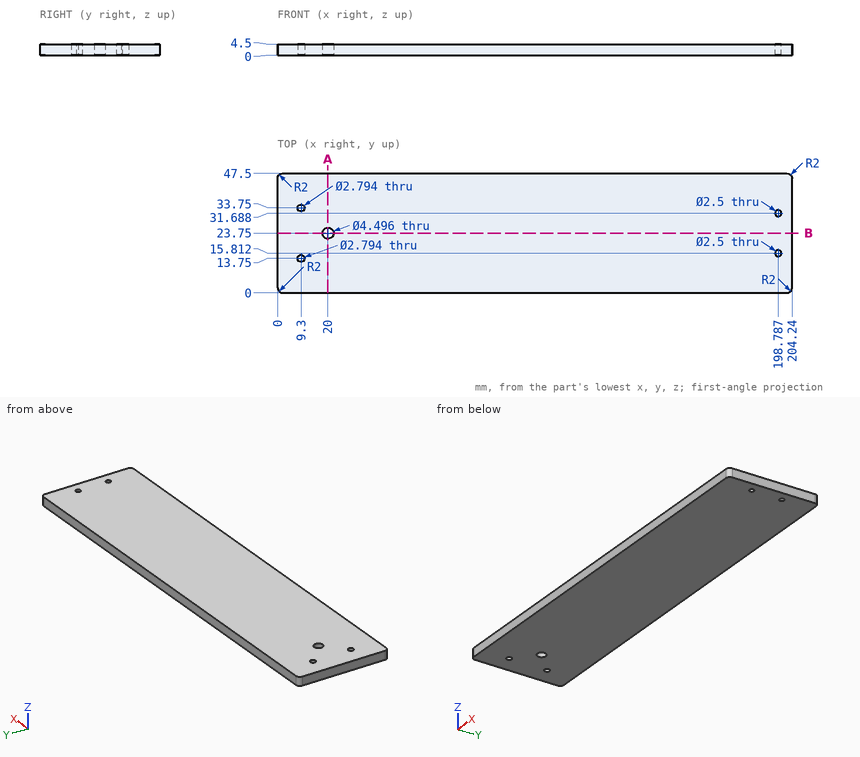
Study the drawing (mm; zero at the part's minimum x, y, z) and answer. Round coordinates to 2 decimals unless told otherwise and drop trailing zeros. Write each loop counter-clockwise with the first axis right and the second up, starting at its lowest first coordinate (ties: lowest second). Pieces come first, ordered by that corner, then holes.
1) A cutting plane is placed at B-B on y = 23.75. Determine the outline of the cut face in (x, z).
2) A cutting plane is placed at A-A on x = 20. Determine the outline of the cut face in (y, z).
3) Consider probe 1 along Y at (x, z) = (9.3, 1.6); probe 2 along X at (y, z) = (15.5, 3.2); probe 3 along X at (y, z) = (34, 1.25) (1 decimal). Determine where each line is inside the solid, lowest interval first.
4) Flat-ended cylindrical pins translate along their axes: P1, Ø2, axis at x = 198.79, y = 31.69, coming from the -Z side; P2, Ø3, axis at x = 9.3, y = 13.75, coming from the -Z side. Find the tip coordinate at first contact, or state that the pin passes through.
Entries:
1. outline: (0, 0) - (17.75, 0) - (17.75, 4.5) - (0, 4.5) - close; (22.25, 0) - (204.24, 0) - (204.24, 4.5) - (22.25, 4.5) - close
2. outline: (0, 0) - (21.5, 0) - (21.5, 4.5) - (0, 4.5) - close; (26, 0) - (47.5, 0) - (47.5, 4.5) - (26, 4.5) - close
3. probe 1: y = 0 to 12.35, 15.15 to 32.35, 35.15 to 47.5
3. probe 2: x = 0 to 197.58, 200 to 204.24
3. probe 3: x = 0 to 7.9, 10.7 to 204.2
4. P1: passes through
4. P2: stops at z = 0
